CAD build for the part. Positions are in the model's coordinates, mm. A direction names the side the tool comes from. Give positions to 0.01 mm unless a question says otherwise; leave off trailing zeros. Loops run counter-clockwise (first coordinate to the right, second up) from the corner with the lowest first, then second, coordinate; pieces in that order, holes last.
Item 1: Saw through at B-B on z = -11.5. Give the cut face in (x, y) (3 decimals), plus the area to 3 significant figures.
Item 2: Probe probe 1 along Y at (x, z) = (-23, -12.5) (3 decimals); probe 2 along Z at (x, y) = (-7, -7.5). List the from-to ranges inside material, lowest first.
Item 3: Saw through at C-C on y = 5. Give the cut face in (x, z).
Item 4: Mould opens along Y. For faces 1 (the flat face through (1, -25.95, -13)), 2 (the flat face through (1, 0, -6.914)), 3 (the flat face through (50.8, -1, -22)) say: released by +Y, released by -Y, zero draft, split by the parting line, or undercut.
Item 5: Which spindle directions (+Z, -Z, +X, -X, +Y, -Y) get a long thin tool onto all of the face, cutting with end or side? Do faces 4 (the flat face through (1, 24.85, -13)), 5 (the flat face through (1, 0, -19.614)). Say none if no direction does.
Item 6: Saw through at A-A on x = 12. Give the cut face in (y, z) (3 decimals).
from build123d import *

# Parameters (mm, degrees)
F0_W     = 50.8
F0_H     = 25.4
F1_DEPTH = 50.8
F2_W     = 19.05
F2_H     = 12.7
F3_DEPTH = 121.595184


with BuildPart() as f1:
    # F0 (on Right) → F1 (new body, symmetric)
    with BuildSketch(Plane.YZ):
        with Locations((-0.54992, -13.264191)):
            Rectangle(F0_W, F0_H)
    extrude(amount=F1_DEPTH, both=True)

    # F2 (on Right) → F3 (cut, symmetric)
    with BuildSketch(Plane.YZ):
        with Locations((0, -13.264191)):
            Rectangle(F2_W, F2_H)
    extrude(amount=F3_DEPTH, both=True, mode=Mode.SUBTRACT)


solid = f1.part
Results below:
1. outline: (-50.8, -25.95) - (50.8, -25.95) - (50.8, -9.525) - (-50.8, -9.525) - close; (-50.8, 9.525) - (50.8, 9.525) - (50.8, 24.85) - (-50.8, 24.85) - close
1. area: 3,230 mm2
2. probe 1: y = -25.95 to -9.525, 9.525 to 24.85
2. probe 2: z = -25.96 to -19.61, -6.91 to -0.56
3. outline: (-50.8, -25.96) - (50.8, -25.96) - (50.8, -19.61) - (-50.8, -19.61) - close; (-50.8, -6.91) - (50.8, -6.91) - (50.8, -0.56) - (-50.8, -0.56) - close
4. face 1: released by -Y
4. face 2: undercut
4. face 3: zero draft
5. face 4: +Z, -Z, +X, -X, +Y
5. face 5: +X, -X
6. outline: (-25.95, -25.964) - (24.85, -25.964) - (24.85, -0.564) - (-25.95, -0.564) - close; hole (-9.525, -19.614) - (9.525, -19.614) - (9.525, -6.914) - (-9.525, -6.914) - close
